from build123d import *

# Parameters (mm, degrees)
SKETCH1_W           = 50
SKETCH1_H           = 20
SKETCH1_R           = 1.75
BOSS_EXTRUDE1_DEPTH = 1.6
SKETCH3_R           = 0.375
CUT_EXTRUDE1_DEPTH  = 2.6
SKETCH2_W           = 0.3
SKETCH2_H           = 20
SKETCH2_W_2         = 1.5
SKETCH2_H_2         = 0.3
CUT_EXTRUDE2_DEPTH  = 0.6
LPATTERN1_COUNT     = 7
LPATTERN1_PITCH     = 5
LPATTERN2_COUNT     = 7
LPATTERN2_PITCH     = 5


with BuildPart() as part:
    # Sketch1 → Boss-Extrude1 (new body)
    with BuildSketch(Plane(origin=(0, 0, 0), x_dir=(1, 0, 0), z_dir=(0, 1, 0))):
        with Locations((25, 10)):
            Rectangle(SKETCH1_W, SKETCH1_H)
        with Locations((3, 17)):
            Circle(SKETCH1_R, mode=Mode.SUBTRACT)
        with Locations((47, 3)):
            Circle(SKETCH1_R, mode=Mode.SUBTRACT)
        with Locations((3, 3)):
            Circle(SKETCH1_R, mode=Mode.SUBTRACT)
        with Locations((47, 17)):
            Circle(SKETCH1_R, mode=Mode.SUBTRACT)
    extrude(amount=BOSS_EXTRUDE1_DEPTH)

    # Sketch3 → Cut-Extrude1 (cut, through all)
    with BuildSketch(Plane(origin=(0, 1.6, 0), x_dir=(1, 0, 0), z_dir=(0, 1, 0))):
        with Locations((8.25, 0.75)):
            Circle(SKETCH3_R)
        with Locations((9.75, 0.75)):
            Circle(SKETCH3_R)
        with Locations((9.75, 5.5)):
            Circle(SKETCH3_R)
        with Locations((9.75, 14.5)):
            Circle(SKETCH3_R)
    cut_extrude1 = extrude(amount=-CUT_EXTRUDE1_DEPTH, mode=Mode.SUBTRACT)

    # Sketch2 → Cut-Extrude2 (cut)
    with BuildSketch(Plane(origin=(0, 1.6, 0), x_dir=(1, 0, 0), z_dir=(0, 1, 0))):
        Polygon((9.15, 0), (9.15, 19.65), (7.5, 19.65), (7.5, 19.35), (8.85, 19.35), (8.85, 0), align=None)
        with Locations((7.5, 10)):
            Rectangle(SKETCH2_W, SKETCH2_H)
        with Locations((10.5, 10)):
            Rectangle(SKETCH2_W, SKETCH2_H)
        with Locations((9.75, 10)):
            Rectangle(SKETCH2_W_2, SKETCH2_H_2)
    cut_extrude2 = extrude(amount=-CUT_EXTRUDE2_DEPTH, mode=Mode.SUBTRACT)

    # LPattern1: Cut-Extrude1 ×7
    with Locations(*[(i * LPATTERN1_PITCH, 0, 0) for i in range(1, LPATTERN1_COUNT)]):
        add(cut_extrude1, mode=Mode.SUBTRACT)

    # LPattern2: Cut-Extrude2 ×7
    with Locations(*[(i * LPATTERN2_PITCH, 0, 0) for i in range(1, LPATTERN2_COUNT)]):
        add(cut_extrude2, mode=Mode.SUBTRACT)


solid = part.part
The listing builds one solid part. Answer for the finished solid, in the listing's coordinates (mm). Coordinates: 2 decimals unless noted, no trailing zeros. Loops run counter-clockwise (first coordinate to the right, second up) from the corner with the lowest first, then second, coordinate; pieces in that order, holes last. Notation, with made-up numbers: (-35, 0.25) -> (-30, 0.25) arc R26 ccw to (-30, 15.25) -> close; hole circle Ø6 at (-34, 71.5). An arc over 180 degrees is marked (long way). Write item = value, one per line. Start each with the question number.
1) The mould has two halves that part along X. Classify faces 1 (the face through (48.669, 0.789, -17.526)), 2 (the face through (9, 1, -10)), 3 (the face through (11, 1.6, -10)): released by +X, released by -X, zero draft, split by the parting line, or undercut.
2) Straight lines are drawn through the part: line 1 (Z direction, x = 23.25, y = 1.25) (3 decimals); line 2 (Z direction, x = 8.25, y = 0.5) (3 decimals); line 3 (Z direction, x = 47, y = 0.95). For each, find the intervals that lie inside material, in ascending order. Write a range as from..to.
3) A cutting plane is placed at A-A (x = 46.5). Give the vertices of the cut face in (y, z), then the cut area to 3 significant figures.
4) Given pin 1 Ø12 at (x, z) = (11.5, -4) entering from -Y, flat-ended and moving along its own axis, determine where the tip first touches the part or whether it passes through.
5) A cutting plane is placed at B-B (z = -17). Count the separate pieces of the cut face and the enclosed holes in it, then the cut area to 3 significant figures.
Responses:
q1.face_1 = undercut
q1.face_2 = undercut
q1.face_3 = zero draft
q2.line_1 = -20..-19.65, -19.35..-1.125, -0.375..0
q2.line_2 = -20..-1.125, -0.375..0
q2.line_3 = -20..-18.75, -15.25..-4.75, -1.25..0
q3.outline = (0, -20) -> (1.6, -20) -> (1.6, -18.68) -> (0, -18.68) -> close; (0, -15.32) -> (1.6, -15.32) -> (1.6, -4.68) -> (0, -4.68) -> close; (0, -1.32) -> (1.6, -1.32) -> (1.6, 0) -> (0, 0) -> close
q3.area = 21.3 mm²
q4.pin_1 = 0
q5.separate_pieces = 3
q5.enclosed_holes = 0
q5.area = 65.0 mm²
